For this review, take the finished solid that the model builds, in its own axes (mm). A direction names the side the tool comes from. Give positions to 0.01 mm unless a question says otherwise; leave off trailing zeros. Order: outer loops, then holes, each group sorted by start corner. A loop starts at its lowest first (then second) coordinate and runs counter-clockwise, first axis right, second up. Notation, with made-up numbers: (-33.5, -19.5) - (-8.5, -19.5) arc R23 ccw to (-8.5, 10.5) - close; hole circle Ø11 at (45, 24). An arc over 180 degrees is marked (long way). Put each result on its own line as item: value. Start each with the question number.
```python
from build123d import *
from build123d.topology import SkipClean

# Parameters (mm, degrees)
BOSS_EXTRUDE1_DEPTH = 23.368
SKETCH4_R           = 49.53
CUT_EXTRUDE1_DEPTH  = 21.59
CUT_EXTRUDE2_START  = -15.24
CUT_EXTRUDE2_DEPTH  = 15.24
BOSS_EXTRUDE2_DEPTH = 15.24
SKETCH8_W           = 12.7
SKETCH8_H           = 2.905378661
BOSS_EXTRUDE3_DEPTH = 2.54
SKETCH9_R           = 0.635
CUT_EXTRUDE4_DEPTH  = 131.041965913


with BuildPart() as part:
    # Sketch1 → Boss-Extrude1 (new body)
    with BuildSketch(Plane.XY):
        with BuildLine():
            Line((0, 0), (12.7, 0))
            Line((12.7, 0), (12.7, 12.7))
            ThreePointArc((12.7, 12.7), (6.35, 113.901562476), (0, 12.7))
            Line((0, 12.7), (0, 0))
        make_face()
    extrude(amount=BOSS_EXTRUDE1_DEPTH)

    # Sketch4 → Cut-Extrude1 (cut)
    with BuildSketch(Plane.XY.offset(23.368)):
        with Locations((6.35, 63.101562476)):
            Circle(SKETCH4_R)
    extrude(amount=-CUT_EXTRUDE1_DEPTH, mode=Mode.SUBTRACT)

    # Sketch5 → Cut-Extrude2 (cut)
    with SkipClean():  # the faces are left unmerged after this step: merging them gives an invalid solid
        with BuildSketch(Plane.XY.offset(23.368).offset(CUT_EXTRUDE2_START)):
            with BuildLine():
                Line((0, 0), (12.7, 0))
                Line((12.7, 0), (12.7, 12.7))
                ThreePointArc((12.7, 12.7), (6.35, 12.301562476), (0, 12.7))
                Line((0, 12.7), (0, 0))
            make_face()
        extrude(amount=CUT_EXTRUDE2_DEPTH, mode=Mode.SUBTRACT)

    # Sketch6 → Boss-Extrude2 (add)
    with BuildSketch(Plane.XY.offset(8.128)):
        with BuildLine():
            Line((12.7, 9.794621339), (0, 9.794621339))
            Line((0, 9.794621339), (0, 12.7))
            ThreePointArc((0, 12.7), (6.35, 12.301562476), (12.7, 12.7))
            Line((12.7, 12.7), (12.7, 9.794621339))
        make_face()
    extrude(amount=BOSS_EXTRUDE2_DEPTH)

    # Sketch8 → Boss-Extrude3 (add)
    with BuildSketch(Plane.XY.offset(23.368)):
        with Locations((6.35, 11.24731067)):
            Rectangle(SKETCH8_W, SKETCH8_H)
    extrude(amount=BOSS_EXTRUDE3_DEPTH)

    # Sketch9 → Cut-Extrude4 (cut, through all)
    with BuildSketch(Plane.ZY):
        with Locations((24.394843598, 11.189256607)):
            Circle(SKETCH9_R)
    extrude(amount=-CUT_EXTRUDE4_DEPTH, mode=Mode.SUBTRACT)


solid = part.part
```
1. Add section C-C, the plane y = 44.5. Give the boundary of the cut face in (x, z).
2. Add section B-B, the plane z = 20. Give the boundary of the cut face in (x, y), then the cut area to 3 significant figures.
3. Add section A-A, the plane x = 6.35. Give the boundary of the cut face in (y, z) (3 decimals).
4. Clearance check with flat-ended pins moving along their axes: pin 1 (8 mm diameter, centred on y = 54, z = 12, fed in from -X); pin 2 (12 mm diameter, centred on y = 28, z = 19, fed in from +X); pin 3 (2 mm diameter, centred on y = 11.19, z = 24.39, fed in from -X). State where each tip first meets the part, or that it passes through.
5. The part is to be moulded in two halves that separate along Y. For faces 6 (the face through (6, 0, 4)), 7 (the face through (6, 11, 25.908)), 8 (the face through (-4.39, 14.75, 12.72)), say which applies: released by +Y, released by -Y, zero draft, split by the parting line, or undercut.
6. Add section D-D, the plane x = 39. Give the boundary of the cut face in (y, z).
7. Wall thickness on line 1 (Z direction, x = 39.5, y = 51.5); line 2 (X direction, y = 93, z = 4.25); line 3 (X direction, y = 61.5, z = 12.75): over which ranges is each line inside the solid? List them lowest first. Write a range as from..to.
8. Tool access review of faces 1 (the face through (0, 8, 7)), 2 (the face through (6, 9.795, 17)), 3 (the face through (6, 12.7, 25)), 4 (the face through (6, 64, 1.778)), 5 (the face through (12.7, 8, 7)): name each direction out of +Z, -Z, +X, -X, +Y, -Y from which nothing blocks a thin tool from reaching the whole face with its end or side.
Found:
1. outline: (-40.92, 0) - (53.62, 0) - (53.62, 23.37) - (52.25, 23.37) - (52.25, 1.78) - (-39.55, 1.78) - (-39.55, 23.37) - (-40.92, 23.37) - close
2. outline: (0, 9.79) - (12.7, 9.79) - (12.7, 12.7) arc R50.8 ccw (long way) to (0, 12.7) - close; hole circle Ø99.06 at (6.35, 63.1)
2. area: 434 mm^2
3. outline: (0, 0) - (113.902, 0) - (113.902, 23.368) - (112.632, 23.368) - (112.632, 1.778) - (13.572, 1.778) - (13.572, 23.368) - (12.7, 23.368) - (12.7, 25.908) - (9.795, 25.908) - (9.795, 8.128) - (0, 8.128) - close; hole circle Ø1.27 at (11.189, 24.395)
4. pin 1: stops at x = -44.19
4. pin 2: stops at x = 47.99
4. pin 3: stops at x = 0
5. face 6: released by -Y
5. face 7: zero draft
5. face 8: undercut
6. outline: (24.18, 0) - (102.02, 0) - (102.02, 23.37) - (100.35, 23.37) - (100.35, 1.78) - (25.86, 1.78) - (25.86, 23.37) - (24.18, 23.37) - close
7. line 1: z = 0..1.78
7. line 2: x = -34.72..-33.14, 45.84..47.42
7. line 3: x = -44.42..-43.15, 55.85..57.12
8. face 1: +Z, -Z, -X, -Y
8. face 2: +Z, +X, -X, -Y
8. face 3: +Z, +X, -X, +Y
8. face 4: +Z
8. face 5: +Z, -Z, +X, -Y
